The model under review builds one solid part; all positions refer to its coordinate system, in mm. Round coordinates to 2 decimals unless told otherwise and drop trailing zeros. Loops run counter-clockwise (first coordinate to the right, second up) from the corner with the lowest first, then second, coordinate; pieces in that order, holes last. Notation, with made-up numbers: (-39.75, -19.75) -> (2.25, -19.75) arc R25 cw to (2.25, 16.25) -> close; hole circle Ø5 at (43.25, 39.25). An arc over 180 degrees is marked (long way). Return JSON: item names as keys, results as strings. Group by question number.
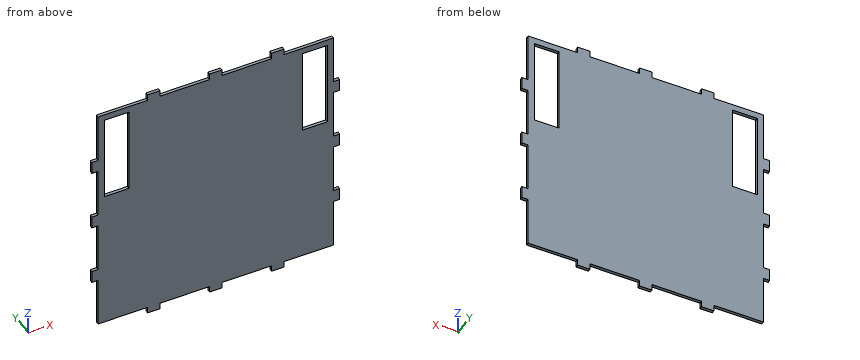
```python
from build123d import *

# Parameters (mm, degrees)
SKETCH1_W           = 12.7
SKETCH1_H           = 44.45
BOSS_EXTRUDE1_DEPTH = 1.5875


with BuildPart() as part:
    # Sketch1 → Boss-Extrude1 (new body)
    with BuildSketch(Plane(origin=(0, 0, 0), x_dir=(1, 0, 0), z_dir=(0, 1, 0))):
        Polygon((3.175, 63.5), (-3.175, 63.5), (-3.175, 60.325), (-28.575, 60.325), (-28.575, 63.5), (-34.925, 63.5), (-34.925, 60.325), (-60.325, 60.325), (-60.325, 34.925), (-63.5, 34.925), (-63.5, 28.575), (-60.325, 28.575), (-60.325, 3.175), (-63.5, 3.175), (-63.5, -3.175), (-60.325, -3.175), (-60.325, -28.575), (-63.5, -28.575), (-63.5, -34.925), (-60.325, -34.925), (-60.325, -60.325), (-34.925, -60.325), (-34.925, -63.5), (-28.575, -63.5), (-28.575, -60.325), (-3.175, -60.325), (-3.175, -63.5), (3.175, -63.5), (3.175, -60.325), (28.575, -60.325), (28.575, -63.5), (34.925, -63.5), (34.925, -60.325), (60.325, -60.325), (60.325, -34.925), (63.5, -34.925), (63.5, -28.575), (60.325, -28.575), (60.325, -3.175), (63.5, -3.175), (63.5, 3.175), (60.325, 3.175), (60.325, 28.575), (63.5, 28.575), (63.5, 34.925), (60.325, 34.925), (60.325, 60.325), (34.925, 60.325), (34.925, 63.5), (28.575, 63.5), (28.575, 60.325), (3.175, 60.325), align=None)
        with Locations((50.8, -34.925)):
            Rectangle(SKETCH1_W, SKETCH1_H, mode=Mode.SUBTRACT)
        with Locations((-50.8, -34.925)):
            Rectangle(SKETCH1_W, SKETCH1_H, mode=Mode.SUBTRACT)
    extrude(amount=BOSS_EXTRUDE1_DEPTH)


solid = part.part
```
1. Wall thickness on line 1 (X direction, y = 0.25, z = 31); line 2 (X direction, y = 0.2, z = 48.5) (3 decimals); line 3 (Z direction, x = -49, y = 1.55) (3 decimals): over which ranges is each line inside the solid? List them lowest first.
2. We need section C-C, the plane x = -39. Write out the cut boundary in (y, z) (1 decimal), then the cut area to 3 significant figures.
3. For P1, Ø0.8, axis at x = -47.5, y = 0.5, coming from the +Z side (3 decimals); P2, Ø0.8, axis at x = -61, y = 1, coming from the +Z side (3 decimals); P3, Ø0.8, axis at x = -44.5, y = 1, coming from the -Z side (3 decimals); P4, Ø10, axis at x = -49.5, z = -36, coming from the -Y side, all flat-tipped, find the tip position at first contact; note any pin that passes through.
4. We need section D-D, the plane z = 7.5. Write out the cut boundary in (x, y) (1 decimal), then the cut area to 3 significant figures.
5. We need section A-A, the plane z = 55.5. Give the number of separate pieces and of enclosed holes in the cut face, then the cut area to 3 significant figures.
Check sheet entries:
{
 "1": {"line 1": "x = -63.5 to -57.15, -44.45 to 44.45, 57.15 to 63.5", "line 2": "x = -60.325 to -57.15, -44.45 to 44.45, 57.15 to 60.325", "line 3": "z = -60.325 to 12.7, 57.15 to 60.325"},
 "2": {"outline": "(0, -60.3) -> (1.6, -60.3) -> (1.6, 60.3) -> (0, 60.3) -> close", "area": "192 mm²"},
 "3": {"P1": "stops at z = 60.325", "P2": "stops at z = 34.925", "P3": "stops at z = -60.325", "P4": "stops at y = 0"},
 "4": {"outline": "(-60.3, 0) -> (60.3, 0) -> (60.3, 1.6) -> (-60.3, 1.6) -> close", "area": "192 mm²"},
 "5": {"separate pieces": "3", "enclosed holes": "0", "area": "151 mm²"}
}
